```python
from build123d import *

# Parameters (mm, degrees)
SKETCH1_W             = 7.62
SKETCH1_H             = 96.52
BOSS_EXTRUDE1_DEPTH   = 7.62
SKETCH2_W             = 7.62
SKETCH2_H             = 5.08
BOSS_EXTRUDE2_DEPTH   = 7.62
SKETCH4_W             = 7.62
SKETCH4_H             = 2.54
BOSS_EXTRUDE3_DEPTH   = 8.128
BOSS_EXTRUDE4_DEPTH   = 2.54
F_6_CLEARANCE_HOLE1_D = 3.7973
CUT_EXTRUDE1_DEPTH    = 2.54
SKETCH12_W            = 7.62
SKETCH12_H            = 25.4
CUT_EXTRUDE2_DEPTH    = 2.54
FILLET2_R             = 12.7
FILLET3_R             = 2.54
SKETCH14_R            = 1.905
CUT_EXTRUDE4_DEPTH    = 99.092682214


with BuildPart() as part:
    # Sketch1 → Boss-Extrude1 (new body)
    with BuildSketch(Plane(origin=(0, 0, 0), x_dir=(0, 0, -1), z_dir=(1, 0, 0))):
        with Locations((3.81, 48.26)):
            Rectangle(SKETCH1_W, SKETCH1_H)
    extrude(amount=BOSS_EXTRUDE1_DEPTH)

    # Sketch2 → Boss-Extrude2 (add)
    with BuildSketch(Plane.ZY):
        with Locations((-3.81, 2.54)):
            Rectangle(SKETCH2_W, SKETCH2_H)
    extrude(amount=BOSS_EXTRUDE2_DEPTH)

    # Sketch4 → Boss-Extrude3 (add)
    with BuildSketch(Plane(origin=(7.62, 0, 0), x_dir=(0, 0, -1), z_dir=(1, 0, 0))):
        with Locations((3.81, 95.25)):
            Rectangle(SKETCH4_W, SKETCH4_H)
    extrude(amount=BOSS_EXTRUDE3_DEPTH)

    # Sketch5 → Boss-Extrude4 (add)
    with BuildSketch(Plane.XZ.offset(-93.98)):
        Polygon((15.748, 0), (12.974546815, -7.62), (10.434546815, -7.62), (13.208, 0), align=None)
    extrude(amount=BOSS_EXTRUDE4_DEPTH)

    # #6 Clearance Hole1 (through all)
    with Locations(Plane(origin=(0, 5.08, 0), x_dir=(1, 0, 0), z_dir=(0, 1, 0))):
        with Locations((-3.81, 3.81)):
            Hole(F_6_CLEARANCE_HOLE1_D / 2)

    # Sketch8 → Cut-Extrude1 (cut)
    with BuildSketch(Plane.XZ.offset(-93.98)):
        Polygon((15.748, -7.62), (12.974546815, -7.62), (15.748, 0), align=None)
    extrude(amount=-CUT_EXTRUDE1_DEPTH, mode=Mode.SUBTRACT)

    # Sketch12 → Cut-Extrude2 (cut)
    with BuildSketch(Plane.ZY):
        with Locations((-3.81, 17.78)):
            Rectangle(SKETCH12_W, SKETCH12_H)
    extrude(amount=-CUT_EXTRUDE2_DEPTH, mode=Mode.SUBTRACT)

    # Fillet2
    # the kernel refuses this fillet: 12.7 mm, written as the material it takes off along each edge
    with BuildSketch(Plane(origin=(0, 30.48, 19.05), x_dir=(1, 0, 0), z_dir=(0, 0, -1))) as fillet2_piece_1:
        with BuildLine():
            CenterArc((12.7, -7.62), FILLET2_R, 143.130102354, 36.869897646)
            Line((0, -7.62), (-0.254, -7.62))
            Line((-0.254, -7.62), (-0.254, 0))
            Line((-0.254, 0), (0, 0.254))
            ThreePointArc((0, 0.254), (1.27, 0.254), (2.3368, 0.1524))
            Line((2.3368, 0.1524), (2.54, 0))
        make_face()
    extrude(amount=45.72, mode=Mode.SUBTRACT)

    # Fillet3
    fillet3_edges = [part.edges().sort_by_distance(p)[0] for p in [
        (2.54, 5.08, -3.81),
        (7.62, 0, -3.81),
        (0, 96.52, -3.81),
    ]]
    fillet(fillet3_edges, radius=FILLET3_R)

    # Sketch14 → Cut-Extrude4 (cut, through all)
    with BuildSketch(Plane.XY):
        with Locations((3.81, 83.82)):
            Circle(SKETCH14_R)
        with Locations((3.81, 44.45)):
            Circle(SKETCH14_R)
        with Locations((3.81, 64.135)):
            Circle(SKETCH14_R)
    extrude(amount=-CUT_EXTRUDE4_DEPTH, mode=Mode.SUBTRACT)


solid = part.part
```
The listing builds one solid part. Answer for the finished solid, in the listing's coordinates (mm). A direction names the side the tool comes from. Coordinates: 2 decimals unless noted, no trailing zeros. Write each loop counter-clockwise with the first axis right and the second up, starting at its lowest first coordinate (ties: lowest second). Pieces come first, ordered by that corner, then holes. Notation, with made-up numbers: (2, -11) - (27, -11) arc R16 ccw to (27, -7) - close; hole circle Ø9 at (51.25, 74.25). An arc over 180 degrees is marked (long way). Return JSON: item names as keys, results as strings. Group by question number.
Q1. Find the intervals of material crossed by line 1 along Y through (x, z) = (3.81, -5) (3 decimals); line 2 along X through (y, z) = (20.5, -0.75); line 3 along Y through (x, z) = (-6.25, -5.75), in increasing order. Write a range as [from, to].
Q2. Which of the six approach directions +Z, -Z, +X, -X, +Y, -Y give full straight-line access (tool end or side, diameter ignored) to faces 1 (the flat face through (-6, 5.08, -5)), 2 (the flat face through (2.54, 19, -4)), 3 (the flat face through (10, 93.98, -4))?
Q3. The part is cut by section B-B on z = -4.75. Write down the section's boundary in (x, y) (3 decimals).
Q4. The part is cut by section C-C on x = -3.81. Write down the section's boundary in (y, z), and give its area (3 significant figures).
Q5. The part is cut by section A-A on y = 83.82. Write down the section's boundary in (x, z) (3 decimals).
Q6. Flat-ended cylindrical pins translate along their axes: pin 1 Ø2 at (y, z) = (44.5, -1.5) entering from +X; pin 2 Ø4 at (y, z) = (19.5, -4.5) entering from -X; pin 3 Ø4 at (x, z) = (-3, -2.5) entering from +Y. Find the tip coordinate at first contact, or state that the pin passes through.
Q7. For a pull along Y with two mould halves and no side action, classify faces 4 (the cylindrical face through (1, 96, -4)), 5 (the cylindrical face through (5.627, 84.392, -3.757)), 6 (the flat face through (13, 91.44, -4)) as +Y half, -Y half, draft (parallel to the pull), parting line (faces both ways), or undercut.
Q8. The part is cut by section D-D on x = 3.81. Write down the section's boundary in (y, z) (3 decimals), and give its area (3 significant figures).
Evaluation:
{
 "1": {"line 1": "y = [0, 42.545], [46.355, 62.23], [66.04, 81.915], [85.725, 96.52]", "line 2": "x = [2.54, 7.62]", "line 3": "y = [0, 5.08]"},
 "2": {"face 1": "+Z, -Z, -X, +Y", "face 2": "+Z, -Z, -X", "face 3": "+Z, -Y"},
 "3": {"outline": "(-7.62, 0) - (-5.46, 0) - (-5.46, 5.08) - (-7.62, 5.08) - close; (-2.16, 0) - (5.08, 0) arc R2.54 ccw to (7.62, 2.54) - (7.62, 93.98) - (11.479, 93.98) - (11.479, 91.44) - (14.019, 91.44) - (14.019, 96.52) - (2.54, 96.52) arc R2.54 ccw to (0, 93.98) - (0, 38.1) arc R12.7 ccw to (2.54, 30.48) - (2.54, 7.62) arc R2.54 cw to (0, 5.08) - (-2.16, 5.08) - close; hole circle Ø3.81 at (3.81, 44.45); hole circle Ø3.81 at (3.81, 64.135); hole circle Ø3.81 at (3.81, 83.82)"},
 "4": {"outline": "(0, -7.62) - (5.08, -7.62) - (5.08, -5.71) - (0, -5.71) - close; (0, -1.91) - (5.08, -1.91) - (5.08, 0) - (0, 0) - close", "area": "19.4 mm2"},
 "5": {"outline": "(0, -7.62) - (1.905, -7.62) - (1.905, 0) - (0, 0) - close; (5.715, -7.62) - (7.62, -7.62) - (7.62, 0) - (5.715, 0) - close"},
 "6": {"pin 1": "stops at x = 7.62", "pin 2": "stops at x = 2.54", "pin 3": "stops at y = 5.08"},
 "7": {"face 4": "+Y half", "face 5": "undercut", "face 6": "-Y half"},
 "8": {"outline": "(0, -7.62) - (42.545, -7.62) - (42.545, 0) - (0, 0) - close; (46.355, -7.62) - (62.23, -7.62) - (62.23, 0) - (46.355, 0) - close; (66.04, -7.62) - (81.915, -7.62) - (81.915, 0) - (66.04, 0) - close; (85.725, -7.62) - (96.52, -7.62) - (96.52, 0) - (85.725, 0) - close", "area": "648 mm2"}
}
